Geometry check sheet. Reference: the model listing, model coordinates, mm. A direction names the side the tool comes from. Round coordinates to 2 decimals unless told otherwise and drop trailing zeros. Write each loop counter-clockwise with the first axis right and the second up, starting at its lowest first coordinate (ties: lowest second). Pieces come first, ordered by that corner, then holes. Notation, with made-up numbers: (42.5, 12.25) - (76.5, 12.25) arc R38 ccw to (76.5, 51.25) - close; hole circle Ø10 at (50.5, 66.25). An arc over 180 degrees is marked (long way). Return JSON: item names as keys, results as strings.
```python
from build123d import *

# Parameters (mm, degrees)
SKETCH2_W           = 25.1
SKETCH2_H           = 57.2
SKETCH2_R           = 1.6
BOSS_EXTRUDE1_DEPTH = 5
BOSS_EXTRUDE2_DEPTH = 6
FILLET1_R           = 2


with BuildPart() as part:
    # Sketch2 → Boss-Extrude1 (new body)
    with BuildSketch(Plane(origin=(0, 0, 0), x_dir=(1, 0, 0), z_dir=(0, 1, 0))):
        with Locations((0, 28.6)):
            Rectangle(SKETCH2_W, SKETCH2_H)
        with Locations((0, 27.6)):
            Circle(SKETCH2_R, mode=Mode.SUBTRACT)
        with Locations((-6.5, 9)):
            Circle(SKETCH2_R, mode=Mode.SUBTRACT)
        with Locations((6.5, 9)):
            Circle(SKETCH2_R, mode=Mode.SUBTRACT)
        with Locations((0, 47.6)):
            Circle(SKETCH2_R, mode=Mode.SUBTRACT)
    boss_extrude1 = extrude(amount=BOSS_EXTRUDE1_DEPTH)

    # Sketch4 → Boss-Extrude2 (add)
    with BuildSketch(Plane(origin=(0, 0, -57.2), x_dir=(-1, 0, 0), z_dir=(0, 0, -1))):
        Polygon((12.55, 0), (-12.55, 0), (-12.55, -10.65), (-7.55, -10.65), (-7.55, -5.65), (7.55, -5.65), (7.55, -10.65), (12.55, -10.65), align=None)
    boss_extrude2 = extrude(amount=-BOSS_EXTRUDE2_DEPTH)

    # Mirror1: Boss-Extrude1, Boss-Extrude2 across plane
    add(boss_extrude1.mirror(Plane.XY))
    add(boss_extrude2.mirror(Plane.XY))

    # Fillet1
    fillet1_edges = [part.edges().sort_by_distance(p)[0] for p in [
        (0, 5, -57.2),
        (0, 5, 57.2),
    ]]
    fillet(fillet1_edges, radius=FILLET1_R)


solid = part.part
```
(1) Gauge pin test, flat end, axial feed: pin 1 (5 mm diameter, centred on x = 0, z = -27.6, fed in from -Y). Record the tip position at first contact, or that the pin passes through.
Response values:
{"pin 1": "stops at y = 0"}
(2) Access from +Z, -Z, +X, -X, +Y, -Y to the whole of each face (thin tool, end or side, straight path). Record for faces 1 (the face through (7.55, -8, -54)), 2 (the face through (0, -4, 51.2)), 3 (the face through (7.24, 2.46, -7.58)).
Response values:
{"face 1": "+Z, -Z, -Y", "face 2": "+X, -X, -Y", "face 3": "+Y, -Y"}
(3) Section check C-C, the plane x = -6.5. Enter the section's corners in (y, z).
Response values:
{"outline": "(-5.65, -57.2) - (3, -57.2) arc R2 ccw to (5, -55.2) - (5, -10.6) - (0, -10.6) - (0, -51.2) - (-5.65, -51.2) - close; (-5.65, 51.2) - (0, 51.2) - (0, 10.6) - (5, 10.6) - (5, 55.2) arc R2 ccw to (3, 57.2) - (-5.65, 57.2) - close; (0, -7.4) - (5, -7.4) - (5, 7.4) - (0, 7.4) - close"}
(4) Section check A-A, the plane y = -1.5. Enter the section's corners in (x, z), plus the area to 3 significant figures.
Response values:
{"outline": "(-12.55, -57.2) - (12.55, -57.2) - (12.55, -51.2) - (-12.55, -51.2) - close; (-12.55, 51.2) - (12.55, 51.2) - (12.55, 57.2) - (-12.55, 57.2) - close", "area": "301 mm^2"}
(5) Section check B-B, the plane z = -27.6. Enter the section's corners in (x, y), plus the area to 4 significant figures.
Response values:
{"outline": "(-12.55, 0) - (-1.6, 0) - (-1.6, 5) - (-12.55, 5) - close; (1.6, 0) - (12.55, 0) - (12.55, 5) - (1.6, 5) - close", "area": "109.5 mm^2"}
(6) Section check D-D, the plane z = 9. Enter the section's corners in (x, y), plus the area to 3 significant figures.
Response values:
{"outline": "(-12.55, 0) - (-8.1, 0) - (-8.1, 5) - (-12.55, 5) - close; (-4.9, 0) - (4.9, 0) - (4.9, 5) - (-4.9, 5) - close; (8.1, 0) - (12.55, 0) - (12.55, 5) - (8.1, 5) - close", "area": "93.5 mm^2"}
(7) Material ranges on line 1 along Z through (x, y) = (0, 2.75); line 2 along X through (y, z) = (3.35, -9); line 3 along Z through (x, y) = (-6.5, 3.15), recorded low to high. Write a range as [from, to].
Response values:
{"line 1": "z = [-57.2, -49.2], [-46, -29.2], [-26, 26], [29.2, 46], [49.2, 57.2]", "line 2": "x = [-12.55, -8.1], [-4.9, 4.9], [8.1, 12.55]", "line 3": "z = [-57.19, -10.6], [-7.4, 7.4], [10.6, 57.19]"}
